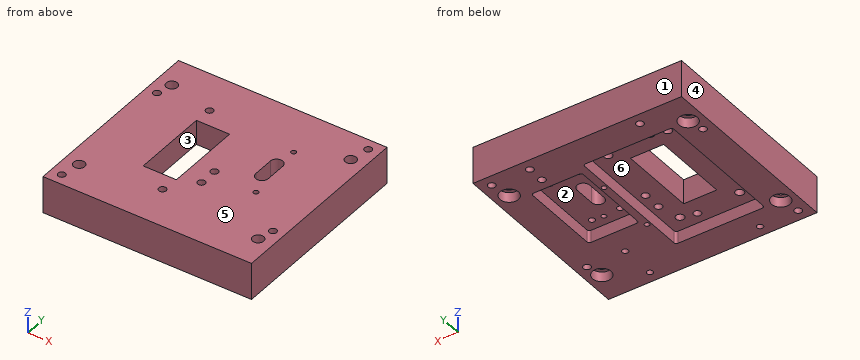
from build123d import *

# Parameters (mm, degrees)
SKETCH2_W                       = 169.5
SKETCH2_H                       = 158
BOSS_EXTRUDE1_DEPTH             = 30
CUT_EXTRUDE2_START              = -10
SKETCH4_R                       = 3.06
SKETCH4_W                       = 27
SKETCH4_H                       = 62
CUT_EXTRUDE2_DEPTH              = 137.360001366
CUT_EXTRUDE4_DEPTH              = 10
SKETCH9_R                       = 2
CUT_EXTRUDE14_DEPTH             = 15
SKETCH11_R                      = 3
CUT_EXTRUDE16_DEPTH             = 7.5
CBORE_FOR_M8_SHCS1_D            = 9
CBORE_FOR_M8_SHCS1_CBORE_D      = 15
CBORE_FOR_M8_SHCS1_CBORE_DEPTH  = 8
M8X1_25_TAPPED_HOLE1_D          = 6.8
M8X1_25_TAPPED_HOLE1_DEPTH      = 12
M8X1_25_TAPPED_HOLE1_TIP        = 2.042926105
M6X1_0_TAPPED_HOLE1_D           = 5
M6X1_0_TAPPED_HOLE1_DEPTH       = 12
M6X1_0_TAPPED_HOLE1_TIP         = 1.502151548
M6X1_0_TAPPED_HOLE2_D           = 5
M6X1_0_TAPPED_HOLE2_DEPTH       = 12
M6X1_0_TAPPED_HOLE2_TIP         = 1.502151548
M6X1_0_TAPPED_HOLE3_D           = 5
M6X1_0_TAPPED_HOLE3_DEPTH       = 12
M6X1_0_TAPPED_HOLE3_CBORE_D     = 6
M6X1_0_TAPPED_HOLE3_CBORE_DEPTH = 6.5
M6X1_0_TAPPED_HOLE3_TIP         = 1.502151548
F_6_0MM_CLEARANCE_DOWEL_HOLE1_D = 6
F_6_0MM_CLEARANCE_DOWEL_HOLE2_D = 6
F_6_0MM_CLEARANCE_DOWEL_HOLE3_D = 6
F_4_0MM_CLEARANCE_DOWEL_HOLE1_D = 4


with BuildPart() as part:
    # Sketch2 → Boss-Extrude1 (new body)
    with BuildSketch(Plane.XY):
        with Locations((-34.75, 0)):
            Rectangle(SKETCH2_W, SKETCH2_H)
    extrude(amount=BOSS_EXTRUDE1_DEPTH)

    # Sketch4 → Cut-Extrude2 (cut, through all)
    with BuildSketch(Plane(origin=(0, 0, 0), x_dir=(-1, 0, 0), z_dir=(0, 0, -1)).offset(CUT_EXTRUDE2_START)):
        with Locations((29, -9)):
            Circle(SKETCH4_R)
        with Locations((29, -24)):
            Circle(SKETCH4_R)
        with BuildLine():
            Line((-5.06, 22), (-5.06, 5))
            ThreePointArc((-5.06, 5), (0, -0.06), (5.06, 5))
            Line((5.06, 5), (5.06, 22))
            ThreePointArc((5.06, 22), (0, 27.06), (-5.06, 22))
        make_face()
        with Locations((58, 0)):
            Rectangle(SKETCH4_W, SKETCH4_H)
    extrude(amount=-CUT_EXTRUDE2_DEPTH, mode=Mode.SUBTRACT)

    # Sketch5 → Cut-Extrude4 (cut)
    with BuildSketch(Plane(origin=(0, 0, 0), x_dir=(-1, 0, 0), z_dir=(0, 0, -1))):
        with BuildLine():
            Line((-25, 45), (-25, -18))
            ThreePointArc((-25, -18), (-24.414213562, -19.414213562), (-23, -20))
            Line((-23, -20), (14, -20))
            ThreePointArc((14, -20), (15.414213562, -19.414213562), (16, -18))
            Line((16, -18), (16, 45))
            ThreePointArc((16, 45), (15.414213562, 46.414213562), (14, 47))
            Line((14, 47), (-23, 47))
            ThreePointArc((-23, 47), (-24.414213562, 46.414213562), (-25, 45))
        make_face()
        with BuildLine():
            Line((24, -54), (92.5, -54))
            ThreePointArc((92.5, -54), (93.914213562, -53.414213562), (94.5, -52))
            Line((94.5, -52), (94.5, 52))
            ThreePointArc((94.5, 52), (93.914213562, 53.414213562), (92.5, 54))
            Line((92.5, 54), (24, 54))
            ThreePointArc((24, 54), (22.585786438, 53.414213562), (22, 52))
            Line((22, 52), (22, -52))
            ThreePointArc((22, -52), (22.585786438, -53.414213562), (24, -54))
        make_face()
    extrude(amount=-CUT_EXTRUDE4_DEPTH, mode=Mode.SUBTRACT)

    # Sketch9 → Cut-Extrude14 (cut)
    with BuildSketch(Plane(origin=(0, 0, 0), x_dir=(-1, 0, 0), z_dir=(0, 0, -1))):
        with Locations((19, 25)):
            Circle(SKETCH9_R)
        with Locations((19, -25)):
            Circle(SKETCH9_R)
    extrude(amount=-CUT_EXTRUDE14_DEPTH, mode=Mode.SUBTRACT)

    # Sketch11 → Cut-Extrude16 (cut)
    with BuildSketch(Plane(origin=(0, 0, 15), x_dir=(-1, 0, 0), z_dir=(0, 0, -1))):
        with Locations((19, 25)):
            Circle(SKETCH11_R)
        with Locations((19, -25)):
            Circle(SKETCH11_R)
    extrude(amount=-CUT_EXTRUDE16_DEPTH, mode=Mode.SUBTRACT)

    # CBORE for M8 SHCS1 (through all)
    with Locations(Plane(origin=(0, 0, 0), x_dir=(-0.9063077870366375, -0.4226182617407263, 0), z_dir=(0, 0, -1))):
        with Locations((74.606700972, 94.372083637), (120.24947324, -3.509157363), (-57.261082041, 32.881126554), (-11.618309773, -65.000114446)):
            CounterBoreHole(CBORE_FOR_M8_SHCS1_D / 2, CBORE_FOR_M8_SHCS1_CBORE_D / 2, CBORE_FOR_M8_SHCS1_CBORE_DEPTH)

    # M8x1.25 Tapped Hole1
    with Locations(Plane(origin=(0, 0, 10), x_dir=(-0.9063077870366375, -0.4226182617407263, 0), z_dir=(0, 0, -1))):
        with Locations((57.020425437, 72.930933649), (13.064497766, 52.433947955), (48.564431752, -23.695906156), (92.520359424, -3.198920462)):
            Hole(M8X1_25_TAPPED_HOLE1_D / 2, depth=M8X1_25_TAPPED_HOLE1_DEPTH)
            with Locations((0, 0, -(M8X1_25_TAPPED_HOLE1_DEPTH + M8X1_25_TAPPED_HOLE1_TIP / 2))):  # 118° drill point
                Cone(0, M8X1_25_TAPPED_HOLE1_D / 2, M8X1_25_TAPPED_HOLE1_TIP, mode=Mode.SUBTRACT)

    # M6x1.0 Tapped Hole1
    with Locations(Plane(origin=(0, 0, 10), x_dir=(-0.9063077870366375, -0.4226182617407263, 0), z_dir=(0, 0, -1))):
        with Locations((-30.560418539, 27.67780372), (10.992955388, -7.011057825), (-9.852123713, -16.731277845), (-9.715339437, 37.39802374)):
            Hole(M6X1_0_TAPPED_HOLE1_D / 2, depth=M6X1_0_TAPPED_HOLE1_DEPTH)
            with Locations((0, 0, -(M6X1_0_TAPPED_HOLE1_DEPTH + M6X1_0_TAPPED_HOLE1_TIP / 2))):  # 118° drill point
                Cone(0, M6X1_0_TAPPED_HOLE1_D / 2, M6X1_0_TAPPED_HOLE1_TIP, mode=Mode.SUBTRACT)

    # M6x1.0 Tapped Hole2
    with Locations(Plane(origin=(0, 0, 0), x_dir=(-0.9063077870366375, -0.4226182617407263, 0), z_dir=(0, 0, -1))):
        with Locations((101.634747391, -29.843393284), (20.520200451, -67.66772771), (8.306532687, -41.475432665)):
            Hole(M6X1_0_TAPPED_HOLE2_D / 2, depth=M6X1_0_TAPPED_HOLE2_DEPTH)
            with Locations((0, 0, -(M6X1_0_TAPPED_HOLE2_DEPTH + M6X1_0_TAPPED_HOLE2_TIP / 2))):  # 118° drill point
                Cone(0, M6X1_0_TAPPED_HOLE2_D / 2, M6X1_0_TAPPED_HOLE2_TIP, mode=Mode.SUBTRACT)

    # M6x1.0 Tapped Hole3
    with Locations(Plane(origin=(0, 0, 0), x_dir=(-0.9063077870366375, -0.4226182617407263, 0), z_dir=(0, 0, -1))):
        with Locations((42.468190748, 97.039696901), (-32.729700528, 46.527053457), (-38.646356192, 59.215362475)):
            CounterBoreHole(M6X1_0_TAPPED_HOLE3_D / 2, M6X1_0_TAPPED_HOLE3_CBORE_D / 2, M6X1_0_TAPPED_HOLE3_CBORE_DEPTH, depth=M6X1_0_TAPPED_HOLE3_DEPTH)
            with Locations((0, 0, -(M6X1_0_TAPPED_HOLE3_DEPTH + M6X1_0_TAPPED_HOLE3_TIP / 2))):  # 118° drill point
                Cone(0, M6X1_0_TAPPED_HOLE3_D / 2, M6X1_0_TAPPED_HOLE3_TIP, mode=Mode.SUBTRACT)

    # Ø6.0mm Clearance Dowel Hole1 (through all)
    with Locations(Plane(origin=(0, 0, 0), x_dir=(-0.9063077870366375, -0.4226182617407263, 0), z_dir=(0, 0, -1))):
        with Locations((-66.74189759, 46.114196361), (82.819661736, 83.857937191)):
            Hole(F_6_0MM_CLEARANCE_DOWEL_HOLE1_D / 2)

    # Ø6.0mm Clearance Dowel Hole2 (through all)
    with Locations(Plane(origin=(0, 0, 0), x_dir=(-0.9063077870366375, -0.4226182617407263, 0), z_dir=(0, 0, -1))):
        with Locations((-19.789008711, -54.576598779), (129.730288789, -16.74222717)):
            Hole(F_6_0MM_CLEARANCE_DOWEL_HOLE2_D / 2)

    # Ø6.0mm Clearance Dowel Hole3 (through all)
    with Locations(Plane(origin=(0, 0, 10), x_dir=(-0.9063077870366375, -0.4226182617407263, 0), z_dir=(0, 0, -1))):
        with Locations((44.876877208, 70.578437869), (60.707979982, -21.343410377)):
            Hole(F_6_0MM_CLEARANCE_DOWEL_HOLE3_D / 2)

    # Ø4.0mm Clearance Dowel Hole1 (through all)
    with Locations(Plane(origin=(0, 0, 10), x_dir=(-0.9063077870366375, -0.4226182617407263, 0), z_dir=(0, 0, -1))):
        with Locations((-18.294727782, 34.500767171), (-1.272735368, -13.834021277)):
            Hole(F_4_0MM_CLEARANCE_DOWEL_HOLE1_D / 2)


solid = part.part
Can you work these out from the model? Positions are in its coordinate system, mm. Face numbers are marked on the shaded views. A direction names the side the tool comes from. Coordinates: 2 decimals unless noted, no trailing zeros.
Q1. If we mould it in two halves opening along X, with no side actions, what happens to the marked faces 4, 5 and 6? For each: +X half, -X half, draft (parallel to the pull), parting line (faces both ways), or undercut.
Results found:
face 4: -X half
face 5: draft
face 6: undercut
Q2. For P1, Ø5.5, axis at x = -29, y = -24, coming from the +Z side; P2, Ø22, axis at x = -54, y = -7.5, coming from the -Z side; P3, Ø13.5, axis at x = -107.5, y = 54, coming from the -Z side; P4, Ø3.5, axis at x = -19, y = -25, coming from the -Z side, each with a flat end and sliding along its axis, tell me the tip position at first contact or that it passes through.
Results found:
P1: passes through
P2: stops at z = 10
P3: stops at z = 8
P4: stops at z = 22.5
Q3. Please list where these lines run through material, in increasing order: L1, parallel to X at y = 15.5, z = 7.75; L2, parallel to Y at x = -70.5, z = 23; L3, parallel to Y at x = -34, z = 18.75.
Results found:
L1: x = -119.5 to -94.5, -22 to -16, 25 to 50
L2: y = -79 to -31, 31 to 42, 48 to 79
L3: y = -79 to -45.4, -38.6 to 38.6, 45.4 to 79
Q4. Which directions (+Z, -Z, +X, -X, +Y, -Y) give clear straight access to the entire face, cutting with the end or side of a thin tool? Please do the marked faces 1, 2 and 3.
Results found:
face 1: +Z, -Z, +X, -X, +Y
face 2: -Z
face 3: +Z, -Z
